Here's how the part is built. I have some questions about the finished solid (model axes, mm). Give positions to 0.01 mm unless a question says otherwise; leave off trailing zeros. Order: outer loops, then holes, each group sorted by start corner. A loop starts at its lowest first (then second) coordinate and runs counter-clockwise, first axis right, second up. Notation, with made-up numbers: (77, 26.5) -> (106, 26.5) arc R25 ccw to (106, 41.5) -> close; hole circle Ø8 at (61, -22.5). An arc over 180 degrees is marked (long way). Write each question's results on one line, items separated by ' | '. Start each with the question number.
Q1. I'm going to push flat-ended pins straight in: pin 1 (12 mm diameter, centred on x = 7.5, y = 33, fed in from -Z); pin 2 (3.5 mm diameter, centred on x = 1.5, y = -35, fed in from -Z). Where does each tip first touch, or does it pass through?
Q2. I need wall thicknesses on line 1 along Z through (x, y) = (-9, -141); line 2 along X through (y, z) = (-126, 6.5); line 3 along X through (y, z) = (-5.5, 11.75). Which ranges of each line are inside material? Lowest first, please. Write a range as [from, to].
Q3. Imagine slicing it at A-A, the plane z = 7. Please give me the cut outline in (x, y).
Q4. Imagine slicing it at B-B, the plane y = 47.5. Please give me the cut outline in (x, z).
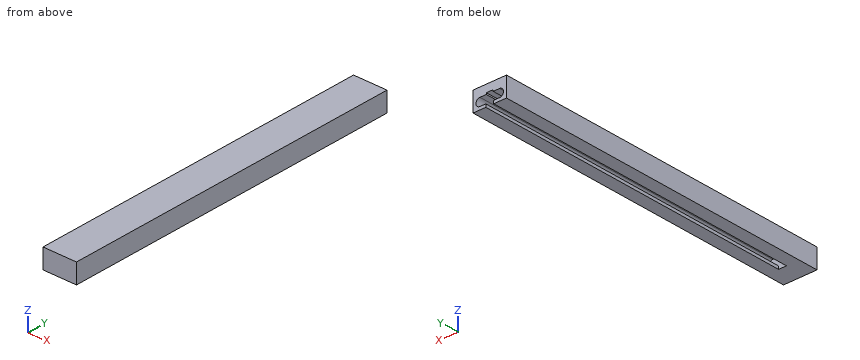
```python
from build123d import *

# Parameters (mm, degrees)
SKETCH1_W           = 34
SKETCH1_H           = 350
BOSS_EXTRUDE1_DEPTH = 20
CUT_EXTRUDE1_DEPTH  = 330


with BuildPart() as part:
    # Sketch1 → Boss-Extrude1 (new body)
    with BuildSketch(Plane.XY):
        Rectangle(SKETCH1_W, SKETCH1_H)
    extrude(amount=BOSS_EXTRUDE1_DEPTH)

    # Sketch2 → Cut-Extrude1 (cut)
    with BuildSketch(Plane(origin=(0, 175, 0), x_dir=(1, 0, 0), z_dir=(0, 1, 0))):
        with BuildLine():
            Line((-10, -3), (-4, -3))
            Line((-4, -3), (-4, 0))
            Line((-4, 0), (4, 0))
            Line((4, 0), (4, -3))
            Line((4, -3), (10, -3))
            ThreePointArc((10, -3), (14, -7), (10, -11))
            Line((10, -11), (3.5, -11))
            Line((3.5, -11), (3.5, -12.5))
            Line((3.5, -12.5), (-3.5, -12.5))
            Line((-3.5, -12.5), (-3.5, -11))
            Line((-3.5, -11), (-10, -11))
            ThreePointArc((-10, -11), (-14, -7), (-10, -3))
        make_face()
    extrude(amount=-CUT_EXTRUDE1_DEPTH, mode=Mode.SUBTRACT)


solid = part.part
```
Geometry check:
1) pin 1: z = 0 | pin 2: z = 12.5
2) line 1: [0, 3], [11, 20] | line 2: [-17, -13.97], [13.97, 17] | line 3: [-17, -3.5], [3.5, 17]
3) outline: (-17, -175) -> (17, -175) -> (17, 175) -> (14, 175) -> (14, -155) -> (-14, -155) -> (-14, 175) -> (-17, 175) -> close
4) outline: (-17, 0) -> (-4, 0) -> (-4, 3) -> (-10, 3) arc R4 cw to (-10, 11) -> (-3.5, 11) -> (-3.5, 12.5) -> (3.5, 12.5) -> (3.5, 11) -> (10, 11) arc R4 cw to (10, 3) -> (4, 3) -> (4, 0) -> (17, 0) -> (17, 20) -> (-17, 20) -> close
